Source: CAD feature listing. Evaluate the final solid. Frame: model axes, mm. Face numbers are marked on the shaded views. A direction names the side the tool comes from. Coordinates: 2 decimals unless noted, no trailing zeros. Order: outer loops, then holes, each group sorted by start corner. A loop starts at its lowest first (then second) coordinate and runs counter-clockwise, first axis right, second up.
Item 1: Reachability of the marked faces 4 and 5 from +Z, -Z, +X, -X, +Y, -Y: full face, straight path, thin tool, end or side. Return the list, or none.
Item 2: Section B-B on y = 0. Return the cut outline in (x, z).
Item 3: Mould query, pull axis Y, two halves, no side actions, for the marked faces 1, 2 and 3. Classes: released by +Y, released by -Y, zero draft, split by the parting line, or undercut.
Item 4: Section D-D on x = 8. Return the cut outline in (y, z), then the cut area to 3 significant figures.
Item 5: Section C-C on x = 0.75. Return the cut outline in (y, z), then the cut area to 3 significant figures.
Item 6: Section A-A on z = 0. Return the cut outline in (x, y), then the cut area to 3 significant figures.
Item 7: Ray query, line 1 (X direction, y = 2.5, z = -2); line 2 (X direction, y = 0.5, z = -1.25); line 3 (X direction, y = 1.25, z = 2). Return the intervals inside material, ascending.
Item 8: Contact query for flat-ended pins moving along their axis: P1, Ø0.7, axis at x = -2.5, z = 0.5, coming from the -Y side; P2, Ø1, axis at x = -2.5, z = -1, coming from the +Y side; P3, Ø5, axis at x = 8.5, y = 0, coming from the -Z side. Output: stop coordinate, or through.
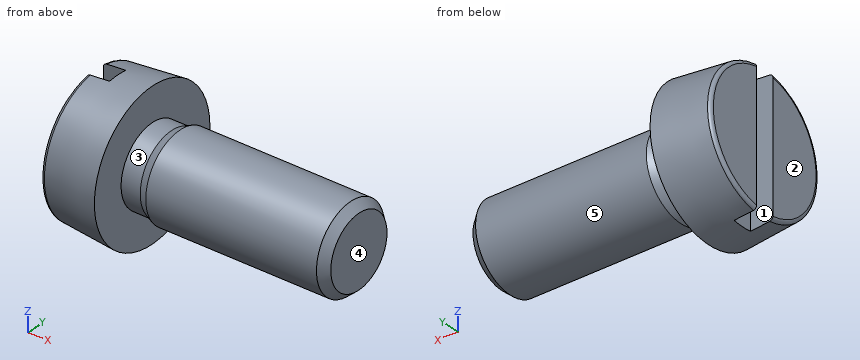
Autodesk Inventor part; units mm, degrees
ref_plane "Work Plane1" through (30.1625, 0, 0) normal (0, 0, -1) x (1, 0, 0)
ref_plane "YZ Plane" through (0, 0, 0) normal (1, 0, 0) x (0, 1, 0)
ref_plane "XZ Plane" through (0, 0, 0) normal (0, 1, 0) x (-1, 0, 0)
sketch "Sketch1" plane through (0, 0, 0) normal (0, 0, 1) x (1, 0, 0)
  line L0 (-3.3, 0) -> (12, 0)
  line L1 (12, 0) -> (12, 2.5)
  line L2 (12, 2.5) -> (1.6, 2.5)
  line L3 (1.6, 2.5) -> (1.1091, 2.2835)
  line L4 (1.1091, 2.2835) -> (0, 2.2835)
  line L5 (0, 2.2835) -> (0, 4.25)
  line L6 (-6.36, 0) -> (15.06, 0)
  line L7 (0, -0.85) -> (0, 5.1)
  line L8 (-3.3, 0) -> (-3.3, 3.9613)
  line L9 (0, 4.25) -> (-3.3, 3.9613)
  line L10 (1.6, 2.5) -> (0, 2.5) construction
  dimension "d0" = 12
  dimension "d1" = 10.4
  dimension "d2" = 0.4909
  dimension "d3" = 3.3
  dimension "d4" = 5
  dimension "d5" = 4.567
  dimension "d9" = 8.5
  dimension "d10" = 5
revolve "Body" add sketch "Sketch1" angle 360 about axis through (-3.3, 0, 0) along (1, 0, 0)
sketch "Sketch2" plane through (-3.3, 0, 0) normal (-1, 0, 0) x (0, 0, 1)
  circle A0 centre (0, 0) radius 4.25
  line L0 (0, 0) -> (0, 3.9613)
  line L1 (-4.25, 0.6) -> (4.25, 0.6)
  line L2 (4.25, 0.6) -> (4.25, -0.6)
  line L3 (4.25, -0.6) -> (-4.25, -0.6)
  line L4 (-4.25, -0.6) -> (-4.25, 0.6)
  line L5 (-4.25, 0) -> (4.25, 0) construction
  line L6 (0, 0.6) -> (0, -0.6) construction
  dimension "d11" = 1.2
  dimension "d12" = 8.5
fillet "Fillet1" radius 0.2 1 edges at (-3.3, -3.9613, 0)
extrude "Slot" cut sketch "Sketch2" against normal blind 1.3 contours A0 L3 L1 | L2 L3 A0 | A0 L1 L2 | A0 L4 L1 | L3 L4 A0
thread "Thread"
chamfer "Chamfer1" distance 0.433 distance2 0.4909 1 edges at (12, -2.5, 0) measured on face at (12, 0.6684, -0.7339)
ref_plane "Work Plane1" through (30.1625, 0, 0) normal (0, 0, -1) x (1, 0, 0)
equation "\"d11\" = SBR"
equation "\"d12\" = KOD"
equation "\"d14\" = RR"
equation "\"d19\" = STI"
equation "\"d15\" = GEL"
equation "\"d17\" = -0.5 * SPD + 0.5 * GD"
equation "\"d0\" = NLG"
equation "\"d1\" = GEL"
equation "\"d3\" = KOH"
equation "\"d4\" = GD"
equation "\"d5\" = BDM"
equation "\"d9\" = KOD"
equation "\"d10\" = KEWI"
equation "\"GD\" = 5"
equation "\"NLG\" = 12"
equation "\"GEL\" = 10.4"
equation "\"KOD\" = 8.5"
equation "\"KOH\" = 3.3"
equation "\"GAL\" = 0.61345 * PTC"
equation "\"SPD\" = 4.13397"
equation "\"BDM\" = 4.56699"
equation "\"GUL\" = 0.61345 * PTC"
equation "\"RR\" = 0.2"
equation "\"SBR\" = 1.2"
equation "\"STI\" = 1.3"
equation "\"KEWI\" = 5deg"
equation "\"PTC\" = 0.8"
equation "\"THREADDIA\" = 5"
equation "\"TOA\" = 30deg"
equation "\"NND\" = 5"
equation "\"GD1\" = THREADDIA - 1.2269 * PTC"
properties part number "DIN 84 - M5 x 12" material "Steel, Mild"
Answer list:
1. face 4: +Z, -Z, +X, +Y, -Y
1. face 5: +X
2. outline: (-2, -4.08) - (0, -4.25) - (0, -2.28) - (1.11, -2.28) - (1.6, -2.5) - (11.51, -2.5) - (12, -2.07) - (12, 2.07) - (11.51, 2.5) - (1.6, 2.5) - (1.11, 2.28) - (0, 2.28) - (0, 4.25) - (-2, 4.08) - close
3. face 1: undercut
3. face 2: zero draft
3. face 3: split by the parting line
4. outline: circle Ø5 at (0, 0)
4. area: 19.6 mm2
5. outline: circle Ø4.57 at (0, 0)
5. area: 16.4 mm2
6. outline: (-3.3, -3.78) arc R0.2 ccw to (-3.12, -3.98) - (0, -4.25) - (0, -2.28) - (1.11, -2.28) - (1.6, -2.5) - (11.51, -2.5) - (12, -2.07) - (12, 2.07) - (11.51, 2.5) - (1.6, 2.5) - (1.11, 2.28) - (0, 2.28) - (0, 4.25) - (-3.12, 3.98) arc R0.2 ccw to (-3.3, 3.78) - (-3.3, 0.6) - (-2, 0.6) - (-2, -0.6) - (-3.3, -0.6) - close
6. area: 84.7 mm2
7. line 1: x = -3.3 to 0
7. line 2: x = -2 to 12
7. line 3: x = -3.3 to 0, 1.28 to 11.67
8. P1: stops at y = -4.05
8. P2: stops at y = 4.01
8. P3: stops at z = -2.5
